Read the model definition and answer for the solid it produces. Units are mm, in the model's axes. Face numbers are marked on the shaded views. A direction names the side the tool comes from. Coordinates: 2 decimals unless noted, no trailing zeros. Loops run counter-clockwise (first coordinate to the right, second up) from the corner with the lowest first, then second, coordinate; pieces in that order, holes last. Notation, with made-up numbers: M 14,26.25 L 48,26.25 A21 ccw 48,38.25 Z; hole C 50,54.25 d4. An arc over 180 degrees is marked long. One line per item, written item: value. Start each with the question number.
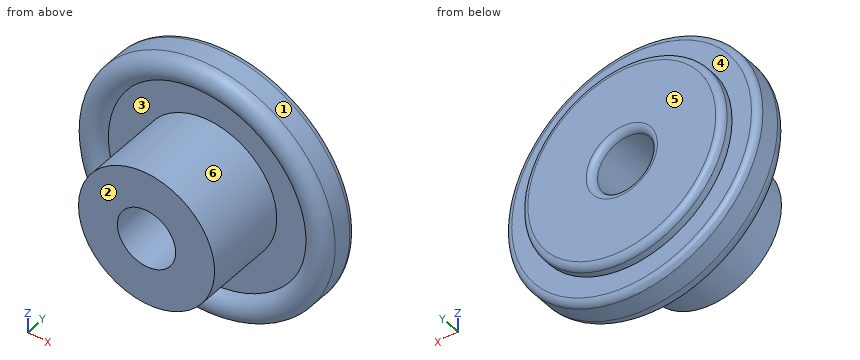
```python
from build123d import *

# Parameters (mm, degrees)
FILLET1_R = 0.5


with BuildPart() as part:
    # Sketch1 → Revolve1 (revolve)
    with BuildSketch(Plane.XY):
        with BuildLine():
            Line((-2.2479, 0), (-2.2479, 9.35))
            Line((-2.2479, 9.35), (-7.7479, 9.35))
            Line((-7.7479, 9.35), (-7.7479, 8.35))
            Line((-7.7479, 8.35), (-9.7479, 8.35))
            Line((-9.7479, 8.35), (-9.7479, 6.35))
            ThreePointArc((-9.7479, 6.35), (-8.7479, 5.35), (-7.7479, 6.35))
            Line((-7.7479, 6.35), (-5.2479, 6.35))
            Line((-5.2479, 6.35), (-5.2479, 0))
            Line((-5.2479, 0), (-2.2479, 0))
        make_face()
    revolve(axis=Axis((0, 0, 0), (0, 1, 0)))

    # Fillet1
    fillet1_edges = [part.edges().sort_by_distance(p)[0] for p in [
        (7.7479, 9.35, 0),
        (2.2479, 9.35, 0),
        (9.7479, 8.35, 0),
    ]]
    fillet(fillet1_edges, radius=FILLET1_R)


solid = part.part
```
1) Section B-B (x = 0) is taken. Determine the outline of the cut face in (y, z).
2) For a pull along Z with two mould halves and no side action, classify the marked faces 1, 2 and 3 as released by +Z, released by -Z, zero draft, split by the parting line, or undercut.
3) Consider line 1 along Z through (x, y) = (0, 5.25); line 2 along Z through (x, y) = (0, 8.75); line 3 along Z through (x, y) = (0.75, 6). Determine where each line is inside the solid, lowest interval first.
4) Section A-A (z = 0) is taken. Determine the outline of the cut face in (x, y), then the cut area to 3 significant figures.
5) Flat-ended cylindrical pins translate along their axes: pin 1 (1.5 mm diameter, centred on y = 7, z = -4, fed in from +X); pin 2 (4 mm diameter, centred on y = 5.5, z = -5, fed in from -X). Find the tip coordinate at first contact, or state that the pin passes through.
6) Section C-C (y = 3.5) is taken. Determine the outline of the cut face in (x, z), then the cut area to 3 significant figures.
7) A tool of negligible diameter and unlimited length cuts with its end or side. For the marked faces 4, 5 and 6, from which of +Z, -Z, +X, -X, +Y, -Y can it reach the whole face along a straight path? Write none if from no direction.
Results found:
1. outline: M 0,-5.25 L 6.35,-5.25 L 6.35,-7.75 A1 ccw 6.35,-9.75 L 7.85,-9.75 A0.5 ccw 8.35,-9.25 L 8.35,-7.75 L 8.85,-7.75 A0.5 ccw 9.35,-7.25 L 9.35,-2.75 A0.5 ccw 8.85,-2.25 L 0,-2.25 Z; M 0,2.25 L 8.85,2.25 A0.5 ccw 9.35,2.75 L 9.35,7.25 A0.5 ccw 8.85,7.75 L 8.35,7.75 L 8.35,9.25 A0.5 ccw 7.85,9.75 L 6.35,9.75 A1 ccw 6.35,7.75 L 6.35,5.25 L 0,5.25 Z
2. face 1: split by the parting line
2. face 2: zero draft
2. face 3: undercut
3. line 1: z = -5.25 to -2.25, 2.25 to 5.25
3. line 2: z = -7.75 to -2.25, 2.25 to 7.75
3. line 3: z = -9.66 to -7.78, -5.19 to -2.12, 2.12 to 5.19, 7.78 to 9.66
4. outline: M -9.75,6.35 A1 ccw -7.75,6.35 L -5.25,6.35 L -5.25,0 L -2.25,0 L -2.25,8.85 A0.5 ccw -2.75,9.35 L -7.25,9.35 A0.5 ccw -7.75,8.85 L -7.75,8.35 L -9.25,8.35 A0.5 ccw -9.75,7.85 Z; M 2.25,0 L 5.25,0 L 5.25,6.35 L 7.75,6.35 A1 ccw 9.75,6.35 L 9.75,7.85 A0.5 ccw 9.25,8.35 L 7.75,8.35 L 7.75,8.85 A0.5 ccw 7.25,9.35 L 2.75,9.35 A0.5 ccw 2.25,8.85 Z
4. area: 81.9 mm²
5. pin 1: stops at x = 9.19
5. pin 2: stops at x = -9.22
6. outline: C 0,0 d10.5; hole C 0,0 d4.5
6. area: 70.6 mm²
7. face 4: +Y
7. face 5: +Z, -Z, +X, -X, +Y
7. face 6: -Y
